Check sheet for the modelled part. Datum: model origin and axes. Units: mm. Give positions to 0.01 mm unless a question says otherwise; leave off trailing zeros. Use CSV: the item, a comma, the result in double quotes. Start each with the question number.
1. Scan lines: line 1 (X direction, y = -0.25, z = 0); line 2 (X direction, y = 1, z = -0.5); line 3 (Z direction, x = 3, y = -4). Record each from-to range of solid material in increasing order.
2. Mould release check, pull along Z, two halves, no side actions. Record for faces 1 (the face through (-51, -5, 0)), 2 (the face through (-2.44, -0.07, -0.54)), 3 (the face through (-50.7, 3.57, 6)), 4 (the face through (-49.3, 3.57, -6)): +Z half, -Z half, draft (parallel to the pull), parting line (faces both ways), or undercut.
3. Cross-section at A-A, the plane z = 0. State how many separate pieces and enclosed holes the cut face has, and give its area (3 significant figures).
4. Depth check by flat-ended pin: P1, Ø3, axis at x = -47.5, z = 5, coming from the +Y side; P2, Ø5, axis at y = -1, z = -3, coming from the +X side; P3, Ø2, axis at x = -80, y = 3.5, coming from the +Z side; P4, Ø6, axis at x = -51, z = -4.5, coming from the +Y side. Enter the tip coordinate at first touch or a pass-through.
from build123d import *

# Parameters (mm, degrees)
CROQUIS1_R              = 2.5
SALIENTE_EXTRUIR1_DEPTH = 5
REDONDEO1_R             = 5


with BuildPart() as part:
    # Croquis1 → Saliente-Extruir1 (new, symmetric)
    with BuildSketch(Plane(origin=(0, 0, 0), x_dir=(-1, 0, 0), z_dir=(0, 1, 0))):
        with BuildLine():
            Line((0, 7.5), (100, 7.5))
            ThreePointArc((100, 7.5), (107.5, 0), (100, -7.5))
            Line((100, -7.5), (0, -7.5))
            ThreePointArc((0, -7.5), (-7.5, 0), (0, 7.5))
        make_face()
        with Locations(Location((0, 0, 0), (0, 0, 90))):
            Circle(CROQUIS1_R, mode=Mode.SUBTRACT)
        with Locations(Location((100, 0, 0), (0, 0, 90))):
            Circle(CROQUIS1_R, mode=Mode.SUBTRACT)
    extrude(amount=SALIENTE_EXTRUIR1_DEPTH, both=True)

    # Redondeo1
    redondeo1_edges = [part.edges().sort_by_distance(p)[0] for p in [
        (7.5, 5, 0),
        (-50, 5, 7.5),
        (-107.5, 5, 0),
        (7.5, -5, 0),
        (-50, -5, 7.5),
        (-107.5, -5, 0),
        (-50, 5, -7.5),
        (-50, -5, -7.5),
    ]]
    fillet(redondeo1_edges, radius=REDONDEO1_R - 0.0001)  # a hair under: the kernel refuses the full size


solid = part.part
Worked answers:
1,line 1,"x = -107.49 to -102.5, -97.5 to -2.5, 2.5 to 7.49"
1,line 2,"x = -107.38 to -102.45, -97.55 to -2.45, 2.45 to 7.38"
1,line 3,"z = -4.61 to 4.61"
2,face 1,"draft"
2,face 2,"undercut"
2,face 3,"+Z half"
2,face 4,"-Z half"
3,separate pieces,"3"
3,enclosed holes,"0"
3,area,"1,030 mm^2"
4,P1,"stops at y = 4.9"
4,P2,"stops at x = 7.47"
4,P3,"stops at z = 6.83"
4,P4,"stops at y = 5"
